Build history of the part. All positions in model axes, mm. A direction names the side the tool comes from. Round coordinates to 2 decimals unless told otherwise and drop trailing zeros. Write each loop counter-clockwise with the first axis right and the second up, starting at its lowest first coordinate (ties: lowest second). Pieces come first, ordered by that corner, then holes. Notation, with made-up numbers: M 84.25,22 L 99.25,22 A27 ccw 99.25,41 Z; hole C 27.5,88.25 d8. An arc over 180 degrees is marked long. Write item = value, one per line. Start each with the question number.
Q1. Probe L1, parallel to X at y = 11.25, z = 5.2; L2, parallel to X at y = -8, z = 1.5; L3, parallel to Y at x = 16.75, z = 4.8. List the from-to ranges inside material, lowest first.
Q2. Band-saw the part on D-D on z = 1. State how many separate pieces and enclosed holes the cut face has, plus the area to 3 significant figures.
Q3. Tool access for faces 1 (the cylindrical face through (18.224, 9.898, 5.028)), 2 (the flat face through (-17, -9, 3)): list every direction of +Z, -Z, +X, -X, +Y, -Y with a clear straight run to the whole face (end or side of a thin tool).
Q4. Pull direction X, two halves, no side cores. Call faces 3 (the cylindrical face through (-25.55, 19.01, 3.79)), 4 (the flat face through (0.32, -20.26, 3.55)), 5 (the cylindrical face through (-11.67, -9.14, 1.48)): released by +X, released by -X, zero draft, split by the parting line, or undercut.
Q5. Band-saw the part on A-A on x = -16.75. Write the cut outline in (y, z).
Q6. Drop flat-ended pins along their axis: P1, Ø1.5, axis at x = 0, z = 4.5, coming from the -Y side; P2, Ø9, axis at x = -16.75, y = -11.25, coming from the -Z side; P3, Ø1.5, axis at x = 16.5, z = 4, coming from the -Y side. Give the stop position or say it passes through.
Q7. Band-saw the part on B-B on y = -11.25. Write the cut outline in (x, z), plus the area to 4 significant figures.
Q8. Band-saw the part on C-C on y = 8. Write the cut outline in (x, z).
```python
from build123d import *

# Parameters (mm, degrees)
F2_DEPTH       = 26.75
F3_R           = 4
F5_D           = 4
F5_DEPTH       = 14.1
F5_CBORE_D     = 11
F5_CBORE_DEPTH = 3
F5_TIP         = 1.2017212381


with BuildPart() as f2:
    # F1 (on Right) → F2 (new body, symmetric)
    with BuildSketch(Plane.YZ):
        Polygon((-19.3, 7), (-21.25, 0), (21.25, 0), (19.3, 7), align=None)
    extrude(amount=F2_DEPTH, both=True)

    # F3
    f3_edges = [f2.edges().sort_by_distance(p)[0] for p in [
        (-26.75, -20.275, 3.5),
        (26.75, -20.275, 3.5),
        (26.75, 20.275, 3.5),
        (-26.75, 20.275, 3.5),
    ]]
    fillet(f3_edges, radius=F3_R)

    # F5
    with Locations(Plane(origin=(0, 0, 0), x_dir=(1, 0, 0), z_dir=(0, 0, -1))):
        with Locations((-16.75, 11.25), (16.75, 11.25), (16.75, -11.25), (-16.75, -11.25)):
            CounterBoreHole(F5_D / 2, F5_CBORE_D / 2, F5_CBORE_DEPTH, depth=F5_DEPTH)
            with Locations((0, 0, -(F5_DEPTH + F5_TIP / 2))):  # 118° drill point
                Cone(0, F5_D / 2, F5_TIP, mode=Mode.SUBTRACT)


solid = f2.part
```
Conclusion:
q1.L1 = -26.75 to -18.75, -14.75 to 14.75, 18.75 to 26.75
q1.L2 = -26.75 to -21.19, -12.31 to 12.31, 21.19 to 26.75
q1.L3 = -19.91 to -13.25, -9.25 to 9.25, 13.25 to 19.91
q2.separate_pieces = 1
q2.enclosed_holes = 4
q2.area = 1,850 mm^2
q3.face_1 = +Z, -Z
q3.face_2 = -Z
q4.face_3 = released by -X
q4.face_4 = zero draft
q4.face_5 = undercut
q5.outline = M -21.25,0 L -16.75,0 L -16.75,3 L -13.25,3 L -13.25,7 L -19.3,7 Z; M -9.25,3 L -5.75,3 L -5.75,0 L 5.75,0 L 5.75,3 L 9.25,3 L 9.25,7 L -9.25,7 Z; M 13.25,3 L 16.75,3 L 16.75,0 L 21.25,0 L 19.3,7 L 13.25,7 Z
q6.P1 = -20.21
q6.P2 = 3
q6.P3 = -20.34
q7.outline = M -26.75,0 L -22.25,0 L -22.25,3 L -18.75,3 L -18.75,7 L -26.75,7 Z; M -14.75,3 L -11.25,3 L -11.25,0 L 11.25,0 L 11.25,3 L 14.75,3 L 14.75,7 L -14.75,7 Z; M 18.75,3 L 22.25,3 L 22.25,0 L 26.75,0 L 26.75,7 L 18.75,7 Z
q7.area = 276.5 mm^2
q8.outline = M -26.75,0 L -21.19,0 L -21.19,3 L -12.31,3 L -12.31,0 L 12.31,0 L 12.31,3 L 21.19,3 L 21.19,0 L 26.75,0 L 26.75,7 L -26.75,7 Z
